Read the model definition and answer for the solid it produces. Units are mm, in the model's axes. A direction names the side the tool comes from. Coordinates: 2 decimals unless noted, no trailing zeros. Order: outer loops, then holes, each group sorted by start corner. A loop starts at its lowest first (then second) coordinate and runs counter-clockwise, first axis right, second up. Notation, with made-up numbers: M 80,-5.5 L 114,-5.5 A25 cw 114,19.5 Z; hole C 34,38 d6. An arc over 180 degrees is marked long. One line per question, with ' | ' between items. Start each with the question number.
1) The mould has two halves that part along Z. Classify faces 3 (the face through (4.93, -9.76, 2.17)), 4 (the face through (4.93, 1.16, -0.55)), 5 (the face through (10, 0, 0)): +Z half, -Z half, draft (parallel to the pull), parting line (faces both ways), or undercut.
2) A tool of negligible diameter and unlimited length cuts with its end or side. For faces 1 (the face through (0, 0, 0)), 2 (the face through (4.93, -0.1, 1.28)), from which of +Z, -Z, +X, -X, +Y, -Y can it reach the whole face along a straight path? Write none if from no direction.
3) Find section A-A, the plane y = 0. Write down the section's boundary in (x, z).
4) Given P1, Ø1, axis at x = 6, y = -3, coming from the +Z side; P2, Ø2, axis at x = 6, y = -8, coming from the -Z side; P3, Ø3, axis at x = 7.5, y = -8, coming from the +Z side, each flat-ended and moving along its own axis, determine where each tip first touches the part or whether it passes through.
5) Find section B-B, the plane x = 5.25. Write down the section's boundary in (y, z), plus the area to 3 significant figures.
6) Find section D-D, the plane z = 8. Write down the section's boundary in (x, y), plus the area to 3 significant figures.
7) Find section C-C, the plane z = -5.25. Write down the section's boundary in (x, y).
8) Consider probe 1 along Z at (x, y) = (3, -3); probe 2 along Z at (x, y) = (2, -3.5); probe 3 along Y at (x, z) = (3.75, -1.25). Determine where each line is inside the solid, lowest interval first.
from build123d import *

# Parameters (mm, degrees)
SKETCH1_R               = 10
BOSS_EXTRUDE1_DEPTH     = 10
CUT_EXTRUDE1_DEPTH      = 18.320508076
CUT_EXTRUDE1_DEPTH_BACK = 18.320508076


with BuildPart() as part:
    # Sketch1 → Boss-Extrude1 (new body)
    with BuildSketch(Plane(origin=(0, 0, 0), x_dir=(0, 0, -1), z_dir=(1, 0, 0))):
        Circle(SKETCH1_R)
    extrude(amount=BOSS_EXTRUDE1_DEPTH)

    # Sketch2 → Cut-Extrude1 (cut, two sides: drawn at the far end of the back side and taken through both)
    with BuildSketch(Plane(origin=(10, 0, 0), x_dir=(0, 0, -1), z_dir=(1, 0, 0)).offset(-CUT_EXTRUDE1_DEPTH_BACK)):
        with BuildLine():
            Line((-6.005338319, 6.239789308), (-1.110102081, 0.645057171))
            ThreePointArc((-1.110102081, 0.645057171), (-1.279247043, -0.109326976), (-0.98454757, -0.824070062))
            Line((-0.98454757, -0.824070062), (-5.632597517, -6.578214359))
            ThreePointArc((-5.632597517, -6.578214359), (-8.656540425, -0.251727641), (-6.005338319, 6.239789308))
        make_face()
        with BuildLine():
            Line((8.406485214, 2.080880889), (1.113686937, 0.638848017))
            ThreePointArc((1.113686937, 0.638848017), (0.544943583, 1.162523924), (-0.221391823, 1.264678237))
            Line((-0.221391823, 1.264678237), (-2.880601988, 8.167079718))
            ThreePointArc((-2.880601988, 8.167079718), (4.110267681, 7.622647737), (8.406485214, 2.080880889))
        make_face()
        with BuildLine():
            Line((-2.401146895, -8.320670197), (-0.003584856, -1.283905188))
            ThreePointArc((-0.003584856, -1.283905188), (0.73430346, -1.053196949), (1.205939393, -0.440608176))
            Line((1.205939393, -0.440608176), (8.513199505, -1.588865359))
            ThreePointArc((8.513199505, -1.588865359), (4.546272744, -7.370920096), (-2.401146895, -8.320670197))
        make_face()
    extrude(amount=CUT_EXTRUDE1_DEPTH + CUT_EXTRUDE1_DEPTH_BACK, mode=Mode.SUBTRACT)


solid = part.part
Report:
1) face 3: parting line | face 4: undercut | face 5: draft
2) face 1: +Z, -Z, -X, +Y, -Y | face 2: +X, -X
3) outline: M 0,-10 L 10,-10 L 10,1.28 L 0,1.28 Z; M 0,8.66 L 10,8.66 L 10,10 L 0,10 Z
4) P1: stops at z = 9.68 | P2: stops at z = -7.14 | P3: stops at z = 7.6
5) outline: C 0,0 d20; hole M -8.32,2.4 A8.66 ccw -1.59,-8.51 L -0.44,-1.21 A1.28 cw -1.28,0 Z; hole M -6.58,5.63 L -0.82,0.98 A1.28 cw 0.65,1.11 L 6.24,6.01 A8.66 ccw Z; hole M 0.64,-1.11 L 2.08,-8.41 A8.66 ccw 8.17,2.88 L 1.26,0.22 A1.28 cw Z | area: 137 mm^2
6) outline: M 0,-6 L 10,-6 L 10,-3.32 L 0,-3.32 Z; M 0,3.32 L 10,3.32 L 10,6 L 0,6 Z | area: 53.7 mm^2
7) outline: M 0,-8.51 L 10,-8.51 L 10,-6.89 L 0,-6.89 Z; M 0,-1.08 L 10,-1.08 L 10,1.46 L 0,1.46 Z; M 0,6.89 L 10,6.89 L 10,8.51 L 0,8.51 Z
8) probe 1: z = -9.54 to -8.12, 0.59 to 2.74, 8.12 to 9.54 | probe 2: z = -9.37 to -7.92, 0.76 to 3.15, 7.92 to 9.37 | probe 3: y = -9.92 to -8.57, -0.45 to 0.67, 8.57 to 9.92
